```python
from build123d import *

# Parameters (mm, degrees)
SKETCH050_R      = 12.4
PAD022_DEPTH     = 20
PAD027_DEPTH     = 8.4
POCKET009_DEPTH  = 12.2
SKETCH057_R      = 6.05
POCKET010_DEPTH  = 3.5
SKETCH058_R      = 5.5
POCKET011_DEPTH  = 4.301
POCKET012_DEPTH  = 28.401
REVOLUTION_ANGLE = 295


with BuildPart() as part:
    # Sketch050 → Pad022 (new body)
    with BuildSketch(Plane.XY.offset(8.4)):
        Circle(SKETCH050_R)
    extrude(amount=PAD022_DEPTH)

    # Sketch049 → Pad027 (join)
    with BuildSketch(Plane.XY):
        with BuildLine():
            ThreePointArc((2.232663, -7.78622), (8.1, 0), (2.232663, 7.78622))
            Line((1.791643, 6.248201), (2.232663, 7.78622))
            ThreePointArc((1.791643, -6.248201), (6.5, 0), (1.791643, 6.248201))
            Line((1.791643, -6.248201), (2.232663, -7.78622))
        make_face()
    extrude(amount=PAD027_DEPTH)

    # Sketch056 → Pocket009 (cut)
    with BuildSketch(Plane(origin=(0, 0, 8.4), x_dir=(1, 0, 0), z_dir=(0, 0, -1))):
        with BuildLine():
            ThreePointArc((2.480736, 8.651355), (-9, 0), (2.480736, -8.651355))
            Line((1.791643, -6.248201), (2.480736, -8.651355))
            ThreePointArc((1.791643, -6.248201), (6.5, 0), (1.791643, 6.248201))
            Line((1.791643, 6.248201), (2.480736, 8.651355))
        make_face()
    extrude(amount=-POCKET009_DEPTH, mode=Mode.SUBTRACT)

    # Sketch057 (on Face10 of Pocket009) → Pocket010 (cut)
    with BuildSketch(Plane(origin=(0, 0, 20.6), x_dir=(1, 0, 0), z_dir=(0, 0, -1))):
        Circle(SKETCH057_R)
    extrude(amount=-POCKET010_DEPTH, mode=Mode.SUBTRACT)

    # Sketch058 → Pocket011 (cut, through all)
    with BuildSketch(Plane(origin=(0, 0, 24.1), x_dir=(1, 0, 0), z_dir=(0, 0, -1))):
        Circle(SKETCH058_R)
    extrude(amount=-POCKET011_DEPTH, mode=Mode.SUBTRACT)

    # Sketch055 (on Face3 of Pocket011) → Pocket012 (cut, through all)
    with BuildSketch(Plane.XY.offset(28.4)):
        with BuildLine():
            ThreePointArc((10.458054, -6.662515), (12.4, 0), (10.458054, 6.662515))
            Line((6.831471, 4.352127), (10.458054, 6.662515))
            ThreePointArc((6.831471, -4.352127), (8.1, 0), (6.831471, 4.352127))
            Line((6.831471, -4.352127), (10.458054, -6.662515))
        make_face()
    extrude(amount=-POCKET012_DEPTH, mode=Mode.SUBTRACT)

    # Sketch059 (on Face5 of Pocket012) → Revolution (revolve)
    with BuildSketch(Plane(origin=(0, 0, 8.4), x_dir=(0.843391, 0.5373, 0), z_dir=(0.5373, -0.843391, 0))):
        with BuildLine():
            Line((12.4, 0), (13.9, 0))
            ThreePointArc((12.4, 3.570696), (12.790231, 1.634214), (13.9, 0))
            Line((12.4, 3.570696), (12.4, 0))
        make_face()
    revolve(axis=Axis((0, 0, 8.4), (0, 0, 1)), revolution_arc=REVOLUTION_ANGLE)


with BuildPart() as part_1:
    # Body006 placement: moved
    add(part.part.moved(Location((0, 0, 2.4))))


solid = part_1.part
```
For this review, take the finished solid that the model builds, in its own axes (mm). A direction names the side the tool comes from. Give positions to 0.01 mm unless a question says otherwise; leave off trailing zeros. Write each loop counter-clockwise with the first axis right and the second up, starting at its lowest first coordinate (ties: lowest second). Pieces come first, ordered by that corner, then holes. Notation, with made-up numbers: M 82.5,-8 L 138.5,-8 A17 ccw 138.5,9 Z; hole C 8.25,-1 d5. An arc over 180 degrees is marked long. Answer as CSV lines item,"result".
1. Draft analysis for pull direction X (two halves, no side actions). For faces 1 (the cylindrical face through (-12.39, 0.45, 22.88)), 2 (the flat face through (10.807, -6.885, 11.8)), 3 (the flat face through (2.01, -7.01, 6.54)), 4 (the cylindrical face through (-1.19, 5.37, 28.62)), state which applies: +X half, -X half, draft (parallel to the pull), parting line (faces both ways), or undercut.
Findings:
face 1,"parting line"
face 2,"+X half"
face 3,"-X half"
face 4,"undercut"
2. For faces 5 (the cylindrical face through (5.589, 2.317, 24.726)), 6 (the flat face through (10.807, 6.885, 11.8)), 7 (the flat face through (2.01, 7.01, 6.54)), 8 (the flat face through (7, 0, 2.4)), list the 3-axis set-ups (+Z, -Z, +X, -X, +Y, -Y) from which the entire face can be reached by the end or side of a thin tool; tool diameter is ignored.
Findings:
face 5,"-Z"
face 6,"+Z, -Z, +X"
face 7,"-Z, -X, +Y"
face 8,"-Z, +X, -X, +Y, -Y"
3. For pin 1 (1 mm diameter, centred on x = 0, z = 23, fed in from +Y); pin 2 (9 mm diameter, centred on x = 0, y = 0, fed in from -Z); pin 3 (12 mm diameter, centred on y = -1, z = 21, fed in from -X); pin 4 (1.5 mm diameter, centred on y = -7, z = 6, fed in from +X), all flat-tipped, find the tip position at first contact; note any pin that passes through.
Findings:
pin 1,"stops at y = 12.4"
pin 2,"passes through"
pin 3,"stops at x = -12.4"
pin 4,"stops at x = 5.15"
4. Consider section A-A, the plane y = 0. Write out the cut boundary in (x, z).
Findings:
outline,"M -13.9,10.8 L -9,10.8 L -9,23 L -6.05,23 L -6.05,26.5 L -5.5,26.5 L -5.5,30.8 L -12.4,30.8 L -12.4,14.37 A5 cw Z; M 5.5,26.5 L 6.05,26.5 L 6.05,23 L 6.5,23 L 6.5,2.4 L 8.1,2.4 L 8.1,30.8 L 5.5,30.8 Z"
5. Consider section B-B, the plane x = 0. Write out the cut boundary in (y, z), then the cut area to 3 significant figures.
Findings:
outline,"M -13.9,10.8 L -9,10.8 L -9,23 L -6.05,23 L -6.05,26.5 L -5.5,26.5 L -5.5,30.8 L -12.4,30.8 L -12.4,14.37 A5 cw Z; M 5.5,26.5 L 6.05,26.5 L 6.05,23 L 9,23 L 9,10.8 L 13.9,10.8 A5 cw 12.4,14.37 L 12.4,30.8 L 5.5,30.8 Z"
area,"190 mm2"
6. Consider section D-D, the plane z = 8.25. Write out the cut boundary in (x, y).
Findings:
outline,"M 1.79,-6.25 L 2.23,-7.79 A8.1 ccw 2.23,7.79 L 1.79,6.25 A6.5 cw Z"
7. Consider section C-C, the plane z = 22.25. Write out the cut boundary in (x, y).
Findings:
outline,"M 6.83,-4.35 A8.1 ccw 6.83,4.35 L 10.46,6.66 A12.4 ccw long 10.46,-6.66 Z; hole M 1.79,-6.25 A6.5 ccw 1.79,6.25 L 2.48,8.65 A9 ccw long 2.48,-8.65 Z"
8. Wall thickness on line 1 (Y direction, x = 0.25, z = 21); line 2 (Y direction, x = 0, z = 28.15); line 3 (Z direction, x = -6.5, y = -2.5): over which ranges is each line inside the solid? List them lowest first.
Findings:
line 1,"y = -12.4 to -9, 9 to 12.4"
line 2,"y = -12.4 to -5.5, 5.5 to 12.4"
line 3,"z = 23 to 30.8"
